from build123d import *

# Parameters (mm, degrees)
SKETCH1_W           = 90
SKETCH1_H           = 30
BOSS_EXTRUDE1_DEPTH = 10
SKETCH3_W           = 10
SKETCH3_H           = 20
BOSS_EXTRUDE2_DEPTH = 11
SKETCH4_R           = 5
BOSS_EXTRUDE3_DEPTH = 10


with BuildPart() as part:
    # Sketch1 → Boss-Extrude1 (new body)
    with BuildSketch(Plane.XY):
        Rectangle(SKETCH1_W, SKETCH1_H)
    extrude(amount=BOSS_EXTRUDE1_DEPTH)

    # Sketch3 → Boss-Extrude2 (add)
    with BuildSketch(Plane(origin=(45, 0, 0), x_dir=(0, 0, -1), z_dir=(1, 0, 0))):
        with Locations((-5, -5)):
            Rectangle(SKETCH3_W, SKETCH3_H)
    boss_extrude2 = extrude(amount=BOSS_EXTRUDE2_DEPTH)

    # Mirror1: Boss-Extrude2 across plane
    add(boss_extrude2.mirror(Plane(origin=(0, 0, 0), x_dir=(0, 0, 1), z_dir=(1, 0, 0))))

    # Sketch4 → Boss-Extrude3 (add)
    with BuildSketch(Plane.XY.offset(10)):
        with Locations(Location((-49, -5, 0), (0, 0, 180))):
            Circle(SKETCH4_R)
    boss_extrude3 = extrude(amount=BOSS_EXTRUDE3_DEPTH)

    # Mirror2: Boss-Extrude3 across plane
    add(boss_extrude3.mirror(Plane(origin=(0, 0, 0), x_dir=(0, 0, 1), z_dir=(1, 0, 0))))


solid = part.part
CAD build for the part. Positions are in the model's coordinates, mm. A direction names the side the tool comes from. Round coordinates to 2 decimals unless told otherwise and drop trailing zeros. Order: outer loops, then holes, each group sorted by start corner. A loop starts at its lowest first (then second) coordinate and runs counter-clockwise, first axis right, second up. Notation, with made-up numbers: (-19, -13) - (3, -13) arc R19 ccw to (3, 6) - close; hole circle Ø7 at (55, 24). An arc over 180 degrees is marked (long way). Return JSON: item names as keys, results as strings.
(1) Wall check: probe 1 along Z at (x, y) = (19, 12.25); probe 2 along X at (y, z) = (11.5, 5); probe 3 along X at (y, z) = (-2.5, 15.25). Give the ranges that are in metal, low to high. Write a range as from..to.
Answer key:
{"probe 1": "z = 0..10", "probe 2": "x = -45..45", "probe 3": "x = -53.33..-44.67, 44.67..53.33"}
(2) Cut at B-B (y = -5). Give the cut face in (x, z).
Answer key:
{"outline": "(-56, 0) - (56, 0) - (56, 10) - (54, 10) - (54, 20) - (44, 20) - (44, 10) - (-44, 10) - (-44, 20) - (-54, 20) - (-54, 10) - (-56, 10) - close"}
(3) Pin check, flat tips, straight feed: pin 1 Ø8 at (x, z) = (-50.5, 5.5) entering from +Y; pin 2 Ø3 at (y, z) = (8.5, 6.5) entering from -X; pin 3 Ø6 at (x, z) = (34, 14.5) entering from +Y. Stop position of each tip, or through.
Answer key:
{"pin 1": "stops at y = 5", "pin 2": "stops at x = -45", "pin 3": "passes through"}
(4) Tool access for faces 1 (the face through (45, 10, 5)), 2 (the face through (-49, -5, 20)), 3 (the face through (-50, 5, 5)): list every direction of +Z, -Z, +X, -X, +Y, -Y with a clear straight run to the whole face (end or side of a thin tool).
Answer key:
{"face 1": "+Z, -Z, +X, +Y", "face 2": "+Z, +X, -X, +Y, -Y", "face 3": "+Z, -Z, -X, +Y"}
(5) Cut at C-C (x = 4.5). Give the cut face in (y, z).
Answer key:
{"outline": "(-15, 0) - (15, 0) - (15, 10) - (-15, 10) - close"}
(6) Cut at D-D (y = -11.25). Give the cut face in (x, z), then the cut area to 3 significant figures.
Answer key:
{"outline": "(-56, 0) - (56, 0) - (56, 10) - (-56, 10) - close", "area": "1,120 mm^2"}
(7) Pull direction X, two halves, no side cores. Call faces 4 (the face through (1, -15, 5)), 5 (the face through (56, -5, 5)), 6 (the face through (45, -2, 15)), 7 (the face through (-45, -2, 15)): +X half, -X half, draft (parallel to the pull), parting line (faces both ways), or undercut.
Answer key:
{"face 4": "draft", "face 5": "+X half", "face 6": "undercut", "face 7": "undercut"}
(8) Cut at A-A (z = 3). Give the cut face in (x, y).
Answer key:
{"outline": "(-56, -15) - (56, -15) - (56, 5) - (45, 5) - (45, 15) - (-45, 15) - (-45, 5) - (-56, 5) - close"}
